Source: CAD feature listing. Evaluate the final solid. Frame: model axes, mm. Face numbers are marked on the shaded views. A direction names the side the tool comes from. Coordinates: 2 decimals unless noted, no trailing zeros. Write each loop counter-clockwise with the first axis right and the second up, starting at its lowest first coordinate (ties: lowest second). Pieces come first, ordered by that corner, then holes. Notation, with made-up numbers: (-20, 34.5) -> (-7, 34.5) arc R8 cw to (-7, 45.5) -> close; hole circle Ø4 at (-29.5, -14). An arc over 180 degrees is marked (long way). Write item = value, one per line.
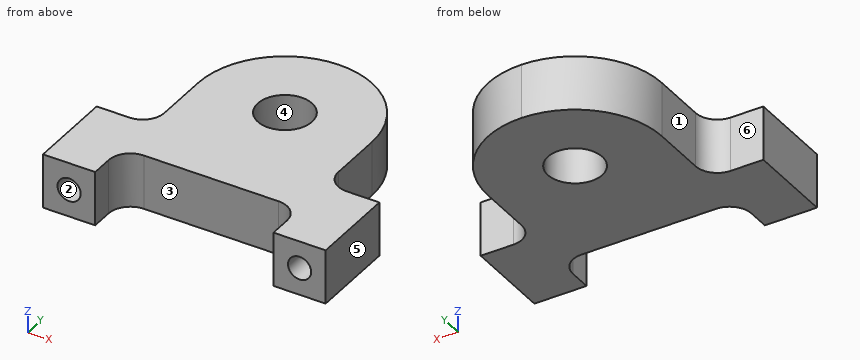
from build123d import *

# Parameters (mm, degrees)
SKETCH1_W                 = 33.02
SKETCH1_H                 = 29.21
BOSS_EXTRUDE1_DEPTH       = 3.175
CUT_EXTRUDE1_REACH        = 24.939
CUT_EXTRUDE2_REACH        = 24.939
SKETCH3_R                 = 3.175
F_6_32_TAPPED_HOLE1_D     = 2.7051
F_6_32_TAPPED_HOLE1_DEPTH = 8.89
F_6_32_TAPPED_HOLE1_TIP   = 0.81269403


with BuildPart() as part:
    # Sketch1 → Boss-Extrude1 (new, symmetric)
    with BuildSketch(Plane.XY):
        Rectangle(SKETCH1_W, SKETCH1_H)
    extrude(amount=BOSS_EXTRUDE1_DEPTH, both=True)

    # Sketch2 → Cut-Extrude1 (cut, up to next)
    with BuildSketch(Plane.XY.offset(3.175), mode=Mode.PRIVATE) as cut_extrude1_sk1:
        with BuildLine():
            Line((-10.16, 4.445), (-10.16, -1.905))
            ThreePointArc((-10.16, -1.905), (-10.903948776, -3.701051224), (-12.7, -4.445))
            Line((-12.7, -4.445), (-16.51, -4.445))
            Line((-16.51, -4.445), (-16.51, 14.605))
            Line((-16.51, 14.605), (0, 14.605))
            ThreePointArc((0, 14.605), (-7.184204897, 11.629204897), (-10.16, 4.445))
        make_face()
    cut_extrude1_tool1 = extrude(cut_extrude1_sk1.sketch, amount=-CUT_EXTRUDE1_REACH, mode=Mode.PRIVATE) & part.part
    # Sketch2 → Cut-Extrude1 (cut, up to next)
    with BuildSketch(Plane.XY.offset(3.175), mode=Mode.PRIVATE) as cut_extrude1_sk2:
        with BuildLine():
            Line((-7.874, -9.525), (0, -9.525))
            Line((0, -9.525), (0, -14.605))
            Line((0, -14.605), (-10.414, -14.605))
            Line((-10.414, -14.605), (-10.414, -12.065))
            ThreePointArc((-10.414, -12.065), (-9.670051224, -10.268948776), (-7.874, -9.525))
        make_face()
    cut_extrude1_tool2 = extrude(cut_extrude1_sk2.sketch, amount=-CUT_EXTRUDE1_REACH, mode=Mode.PRIVATE) & part.part
    cut_extrude1_1 = cut_extrude1_tool1.solids().sort_by_distance((-12.509542, 6.301506, 3.175))[0]
    add(cut_extrude1_1, mode=Mode.SUBTRACT)
    cut_extrude1_2 = cut_extrude1_tool2.solids().sort_by_distance((-5.082313, -12.118013, 3.175))[0]
    add(cut_extrude1_2, mode=Mode.SUBTRACT)
    cut_extrude1 = cut_extrude1_1 + cut_extrude1_2  # Cut-Extrude1 as one shape, for the pattern or mirror that repeats it

    # Mirror1: Cut-Extrude1 across plane
    add(cut_extrude1.mirror(Plane(origin=(0, 0, 0), x_dir=(0, 0, 1), z_dir=(1, 0, 0))), mode=Mode.SUBTRACT)

    # Sketch3 → Cut-Extrude2 (cut, up to next)
    with BuildSketch(Plane.XY.offset(3.175), mode=Mode.PRIVATE) as cut_extrude2_sk1:
        with Locations((0, 4.445)):
            Circle(SKETCH3_R)
    cut_extrude2_tool1 = extrude(cut_extrude2_sk1.sketch, amount=-CUT_EXTRUDE2_REACH, mode=Mode.PRIVATE) & part.part
    add(cut_extrude2_tool1.solids().sort_by_distance((0, 4.445, 3.175))[0], mode=Mode.SUBTRACT)

    # #6-32 Tapped Hole1
    with Locations(Plane(origin=(0, -14.605, 0), x_dir=(-1, 0, 0), z_dir=(0, -1, 0))):
        with Locations((-13.462, 0), (13.462, 0)):
            Hole(F_6_32_TAPPED_HOLE1_D / 2, depth=F_6_32_TAPPED_HOLE1_DEPTH)
            with Locations((0, 0, -(F_6_32_TAPPED_HOLE1_DEPTH + F_6_32_TAPPED_HOLE1_TIP / 2))):  # 118° drill point
                Cone(0, F_6_32_TAPPED_HOLE1_D / 2, F_6_32_TAPPED_HOLE1_TIP, mode=Mode.SUBTRACT)


solid = part.part
1) Cut plane C-C, the plane y = -1.25. Output: boundary loops of the cut face in (x, z) (3 decimals), and give its area (3 significant figures).
Answer block:
outline = (-10.16, -3.175) -> (10.16, -3.175) -> (10.16, 3.175) -> (-10.16, 3.175) -> close
area = 129 mm2
2) Reachability of the marked faces 1, 2 and 3 from +Z, -Z, +X, -X, +Y, -Y: full face, straight path, thin tool, end or side. Return the list, or none.
Answer block:
face_1 = +Z, -Z, -X, +Y
face_2 = -Y
face_3 = +Z, -Z, -Y
3) Cut plane A-A, the plane z = -2.75. Output: boundary loops of the cut face in (x, y) (3 decimals), and give its area (3 significant figures).
Answer block:
outline = (-16.51, -14.605) -> (-10.414, -14.605) -> (-10.414, -12.065) arc R2.54 cw to (-7.874, -9.525) -> (7.874, -9.525) arc R2.54 cw to (10.414, -12.065) -> (10.414, -14.605) -> (16.51, -14.605) -> (16.51, -4.445) -> (12.7, -4.445) arc R2.54 cw to (10.16, -1.905) -> (10.16, 4.445) arc R10.16 ccw to (-10.16, 4.445) -> (-10.16, -1.905) arc R2.54 cw to (-12.7, -4.445) -> (-16.51, -4.445) -> close; hole circle Ø6.35 at (0, 4.445)
area = 546 mm2
4) Material intervals for probe 1 along Y at (x, z) = (0, 1.75) (3 decimals); probe 2 along Y at (x, z) = (15, 0) (3 decimals); probe 3 along X at (y, z) = (-12.5, 1.75), sorted ascending. Write a range as [from, to].
Answer block:
probe_1 = [-9.525, 1.27], [7.62, 14.605]
probe_2 = [-14.605, -4.445]
probe_3 = [-16.51, -10.41], [10.41, 16.51]
5) Cut plane B-B, the plane y = -8. Output: boundary loops of the cut face in (x, z) (3 decimals), and give its area (3 significant figures).
Answer block:
outline = (-16.51, -3.175) -> (16.51, -3.175) -> (16.51, 3.175) -> (-16.51, 3.175) -> close; hole circle Ø2.705 at (-13.462, 0); hole circle Ø2.705 at (13.462, 0)
area = 198 mm2
6) First-contact query: pin 1 Ø10 at (x, y) = (0, 4.445) entering from -Z (3 decimals); pin 2 Ø2 at (x, z) = (-13.462, 0) entering from -Y; pin 3 Ø2 at (x, z) = (6.5, -2.5) entering from -Y (3 decimals); pin 4 Ø1.1 at (x, z) = (14, -0.5) entering from +Y (3 decimals). Flat tips, straight axial feed; report the tip coordinate or a pass-through.
Answer block:
pin_1 = -3.175
pin_2 = -5.5
pin_3 = -9.525
pin_4 = -4.445
7) Pull-direction query (Y, two-part tool) for the marked faces 4, 5 and 6; classes: +Y half, -Y half, draft (parallel to the pull), parting line (faces both ways), or undercut.
Answer block:
face_4 = undercut
face_5 = draft
face_6 = +Y half
8) Cut plane D-D, the plane x = 4. Output: boundary loops of the cut face in (y, z) (3 decimals).
Answer block:
outline = (-9.525, -3.175) -> (13.784, -3.175) -> (13.784, 3.175) -> (-9.525, 3.175) -> close
